```python
from build123d import *

# Parameters (mm, degrees)
SKETCH8_W           = 10.392304846
SKETCH8_H           = 6
BOSS_EXTRUDE3_DEPTH = 5.5
CUT_EXTRUDE5_DEPTH  = 11.392304845
CUT_EXTRUDE7_REACH  = 8
SKETCH11_R          = 0.925
CUT_EXTRUDE8_REACH  = 4.25
SKETCH12_R          = 1.05
CUT_EXTRUDE6_DEPTH  = 7


with BuildPart() as part:
    # Sketch8 → Boss-Extrude3 (new body)
    with BuildSketch(Plane.XY):
        Rectangle(SKETCH8_W, SKETCH8_H)
    extrude(amount=BOSS_EXTRUDE3_DEPTH)

    # Sketch9 → Cut-Extrude5 (cut, through all)
    with BuildSketch(Plane(origin=(5.196152423, 0, 0), x_dir=(0, 0, -1), z_dir=(1, 0, 0))):
        with BuildLine():
            Line((-1.702049043, 0.75), (-5.5, 0.75))
            Line((-5.5, 0.75), (-5.5, -0.75))
            Line((-5.5, -0.75), (-1.702049043, -0.75))
            ThreePointArc((-1.702049043, -0.75), (-0.5, 0), (-1.702049043, 0.75))
        make_face()
    extrude(amount=-CUT_EXTRUDE5_DEPTH, mode=Mode.SUBTRACT)

    # Sketch11 → Cut-Extrude7 (cut, up to next)
    with BuildSketch(Plane(origin=(0, 3, 0), x_dir=(1, 0, 0), z_dir=(0, 1, 0)), mode=Mode.PRIVATE) as cut_extrude7_sk1:
        with Locations((0, -3.5)):
            Circle(SKETCH11_R)
    cut_extrude7_tool1 = extrude(cut_extrude7_sk1.sketch, amount=-CUT_EXTRUDE7_REACH, mode=Mode.PRIVATE) & part.part
    add(cut_extrude7_tool1.solids().sort_by_distance((0, 3, 3.5))[0], mode=Mode.SUBTRACT)

    # Sketch12 → Cut-Extrude8 (cut, up to next)
    with BuildSketch(Plane(origin=(0, -0.75, 0), x_dir=(1, 0, 0), z_dir=(0, 1, 0)), mode=Mode.PRIVATE) as cut_extrude8_sk1:
        with Locations((0, -3.5)):
            Circle(SKETCH12_R)
    cut_extrude8_tool1 = extrude(cut_extrude8_sk1.sketch, amount=-CUT_EXTRUDE8_REACH, mode=Mode.PRIVATE) & part.part
    add(cut_extrude8_tool1.solids().sort_by_distance((0, -0.75, 3.5))[0], mode=Mode.SUBTRACT)

    # Sketch10 → Cut-Extrude6 (cut, through all)
    with BuildSketch(Plane.XZ.offset(3)):
        Polygon((5.196152423, 0), (3.194316134, 5.5), (5.196152423, 5.5), align=None)
        Polygon((-5.196152423, 5.5), (-5.196152423, 0), (-3.194316134, 5.5), align=None)
    extrude(amount=-CUT_EXTRUDE6_DEPTH, mode=Mode.SUBTRACT)


solid = part.part
```
Check sheet for the modelled part. Datum: model origin and axes. Units: mm. A direction names the side the tool comes from. Coordinates: 2 decimals unless noted, no trailing zeros. Loops run counter-clockwise (first coordinate to the right, second up) from the corner with the lowest first, then second, coordinate; pieces in that order, holes last.
1) Sectioned sample at B-B (z = 4.25). Record the boundary of the cut face in (x, y).
2) Release check for a two-part mould opening along Z. For faces 4 (the face through (0, -3, 2)), 5 (the face through (0, 2, 5.5)), 6 (the face through (0.1, 0, 0.5)) record: released by +Z, released by -Z, zero draft, split by the parting line, or undercut.
3) Sectioned sample at D-D (z = 4.85). Record the boundary of the cut face in (x, y).
4) Gauge pin test, flat ends, axial feed: pin 1 (2.5 mm diameter, centred on x = 0, z = 3.5, fed in from -Y); pin 2 (1.7 mm diameter, centred on x = 0, z = 3.5, fed in from -Y); pin 3 (1 mm diameter, centred on y = -1, z = 1.5, fed in from -X); pin 4 (2.5 mm diameter, centred on y = 0, z = 1.335, fed in from -X). Record the tip position at first contact, or that the pin passes through.
5) Access from +Z, -Z, +X, -X, +Y, -Y to the whole of each face (thin tool, end or side, straight path). Record for faces 1 (the face through (-0.14, -1.86, 2.46)), 2 (the face through (0, -0.75, 2)), 3 (the face through (-0.12, 1.891, 2.583)).
6) Material ranges on probe 1 along Y at (x, z) = (2, 2.5); probe 2 along Z at (x, y) = (0, -1.55); probe 3 along Z at (x, y) = (0, 1.7) (3 decimals), recorded low to high.
7) Sectioned sample at C-C (x = -2.25). Record the boundary of the cut face in (y, z) (3 decimals).
8) Sectioned sample at A-A (x = 0). Record the boundary of the cut face in (y, z) (3 decimals), and give its area (3 significant figures).
Check sheet entries:
1. outline: (-3.65, -3) - (-0.73, -3) - (-0.73, -0.75) - (-3.65, -0.75) - close; (-3.65, 0.75) - (-0.54, 0.75) - (-0.54, 3) - (-3.65, 3) - close; (0.54, 0.75) - (3.65, 0.75) - (3.65, 3) - (0.54, 3) - close; (0.73, -3) - (3.65, -3) - (3.65, -0.75) - (0.73, -0.75) - close
2. face 4: zero draft
2. face 5: released by +Z
2. face 6: undercut
3. outline: (-3.43, -3) - (3.43, -3) - (3.43, -0.75) - (-3.43, -0.75) - close; (-3.43, 0.75) - (3.43, 0.75) - (3.43, 3) - (-3.43, 3) - close
4. pin 1: stops at y = -3
4. pin 2: passes through
4. pin 3: stops at x = -4.83
4. pin 4: stops at x = -5.17
5. face 1: -Y
5. face 2: +Z, +X, -X
5. face 3: +Y, -Y
6. probe 1: y = -3 to -0.75, 0.75 to 3
6. probe 2: z = 0 to 2.45, 4.55 to 5.5
6. probe 3: z = 0 to 2.575, 4.425 to 5.5
7. outline: (-3, 0) - (3, 0) - (3, 5.5) - (0.75, 5.5) - (0.75, 1.702) arc R0.835 cw (long way) to (-0.75, 1.702) - (-0.75, 5.5) - (-3, 5.5) - close
8. outline: (-3, 0) - (3, 0) - (3, 2.575) - (0.75, 2.575) - (0.75, 1.702) arc R0.835 cw (long way) to (-0.75, 1.702) - (-0.75, 2.45) - (-3, 2.45) - close; (-3, 4.55) - (-0.75, 4.55) - (-0.75, 5.5) - (-3, 5.5) - close; (0.75, 4.425) - (3, 4.425) - (3, 5.5) - (0.75, 5.5) - close
8. area: 16.7 mm2
